```python
from build123d import *

# Parameters (mm, degrees)
SKETCH1_R           = 6
BOSS_EXTRUDE1_DEPTH = 40
BOSS_EXTRUDE2_DEPTH = 1.3
BOSS_EXTRUDE3_START = -0.085027
BOSS_EXTRUDE3_DEPTH = 0.085027


with BuildPart() as part:
    # Sketch1 → Boss-Extrude1 (new body)
    with BuildSketch(Plane.XY):
        Circle(SKETCH1_R)
    extrude(amount=-BOSS_EXTRUDE1_DEPTH)



with BuildPart() as body_2:
    # Sketch3 → Boss-Extrude2 (new body)
    with BuildSketch(Plane(origin=(0, 6, 0), x_dir=(-1, 0, 0), z_dir=(0, 1, 0))):
        Polygon((0, -14.998657747), (-1.006524795, -14.998657747), (-1.006524795, -26.292665591), (0, -26.292665591), (1.006524795, -26.292665591), (1.006524795, -14.998657747), align=None)
    extrude(amount=BOSS_EXTRUDE2_DEPTH)


with BuildPart() as part_1:
    add(part.part)

    add(body_2.part)  # Boss-Extrude3 merges body 2
    # Sketch3<2> → Boss-Extrude3 (add)
    with BuildSketch(Plane(origin=(0, 6, 0), x_dir=(-1, 0, 0), z_dir=(0, 1, 0)).offset(BOSS_EXTRUDE3_START)):
        Polygon((0, -14.998657747), (-1.006524795, -14.998657747), (-1.006524795, -26.292665591), (0, -26.292665591), (1.006524795, -26.292665591), (1.006524795, -14.998657747), align=None)
    extrude(amount=BOSS_EXTRUDE3_DEPTH)


solid = part_1.part
```
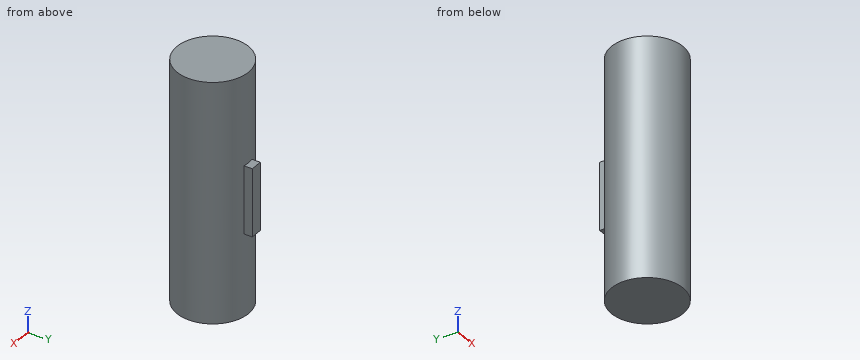
For this review, take the finished solid that the model builds, in its own axes (mm). Coordinates: 2 decimals unless noted, no trailing zeros. Loops run counter-clockwise (first coordinate to the right, second up) from the corner with the lowest first, then second, coordinate; pieces in that order, holes last. Notation, with made-up numbers: (29.25, 19) - (46.25, 19) arc R12 ccw to (46.25, 25) - close; hole circle Ø8 at (88, 74.25). An arc over 180 degrees is marked (long way). Use one line per item in the form item = value. Start each with the question number.
1) To check wall thickness, follow probe 1 along X at (y, z) = (5.5, -26.5); probe 2 along Y at (x, z) = (-2.75, -20); probe 3 along Y at (x, z) = (-1.5, -1.5). State the ranges of each line that lie inside material, in increasing order. Write a range as from..to.
2) Take a section at D-D (z = -24). State the section outline as (x, y) points, plus the area to 3 significant figures.
3) Take a section at B-B (z = -34.5). State the section outline as (x, y) points, plus the area to 3 significant figures.
4) Take a section at C-C (y = 5). State the section outline as (x, z) points.
5) For pin 1 (1 mm diameter, centred on y = -3.5, z = -18.5, fed in from -X); pin 2 (1.1 mm diameter, centred on y = 6.5, z = -20, fed in from +X); pin 3 (1.5 mm diameter, centred on x = 0, y = 7, fed in from -Z), all flat-tipped, find the tip position at first contact; note any pin that passes through.
6) Take a section at A-A (x = 0). State the section outline as (y, z) points.
From the geometry:
q1.probe_1 = -2.4..2.4
q1.probe_2 = -5.33..5.33
q1.probe_3 = -5.81..5.81
q2.outline = (-1.01, 5.91) arc R6 ccw (long way) to (1.01, 5.91) - (1.01, 7.3) - (-1.01, 7.3) - close
q2.area = 116 mm2
q3.outline = circle Ø12 at (0, 0)
q3.area = 113 mm2
q4.outline = (-3.32, -40) - (3.32, -40) - (3.32, 0) - (-3.32, 0) - close
q5.pin_1 = -5.2
q5.pin_2 = 1.01
q5.pin_3 = -26.29
q6.outline = (-6, -40) - (6, -40) - (6, -26.29) - (7.3, -26.29) - (7.3, -15) - (6, -15) - (6, 0) - (-6, 0) - close
